Job drawing, mm, ordinate dimensions from the low corner. One solid piece. A direction names the side the tool comes from. Give positions to 0.01 mm unless a question says otherwise; leave off trailing zeros. Order: outer loops, then holes, each group sorted by start corner. A loop starts at its lowest first (then second) coordinate and runs counter-clockwise, first axis right, second up. Notation, with made-up numbers: M -12,14.5 L 37,14.5 A27 cw 37,50.5 Z; hole C 59.5,66 d10. An arc over 180 degrees is marked long. Put each result on its own line as item: value. Start each with the question number.
1) Drill centre lines: line 1 (Z direction, x = 11, y = 0.35); line 2 (Z direction, x = 11, y = 2.25); line 3 (Z direction, x = 13.5, y = 1.75). Where is each one in solid material? Low to high. Write a range as [from, to].
2) Cut at D-D (z = 19). Write the cut outline in (x, y), and give its area (3 significant figures).
3) Tool access for the marked faces 1, 2 and 3: list every direction of +Z, -Z, +X, -X, +Y, -Y with a clear straight run to the whole face (end or side of a thin tool).
4) Pin check, flat tips, straight feed: pin 1 (3 mm diameter, centred on x = 19, y = 3, fed in from -Z); pin 2 (1 mm diameter, centred on x = 5, y = 4, fed in from -Z); pin 3 (9.5 mm diameter, centred on x = 10, z = 7.5, fed in from +Y); pin 4 (4 mm diameter, centred on x = 8, y = 3, fed in from -Z). Stop position of each tip, or through.
5) Two-plate mould, pull along Z, no slides. Class the marked faces 4, 5 and 6: released by +Z, released by -Z, zero draft, split by the parting line, or undercut.
6) Cut at B-B (z = 11). Write the cut outline in (x, y), and give its area (3 significant figures).
7) Cut at A-A (x = 11). Write the cut outline in (y, z), and give its area (3 significant figures).
8) Cut at C-C (y = 4.75). Write the cut outline in (x, z), and give its area (3 significant figures).
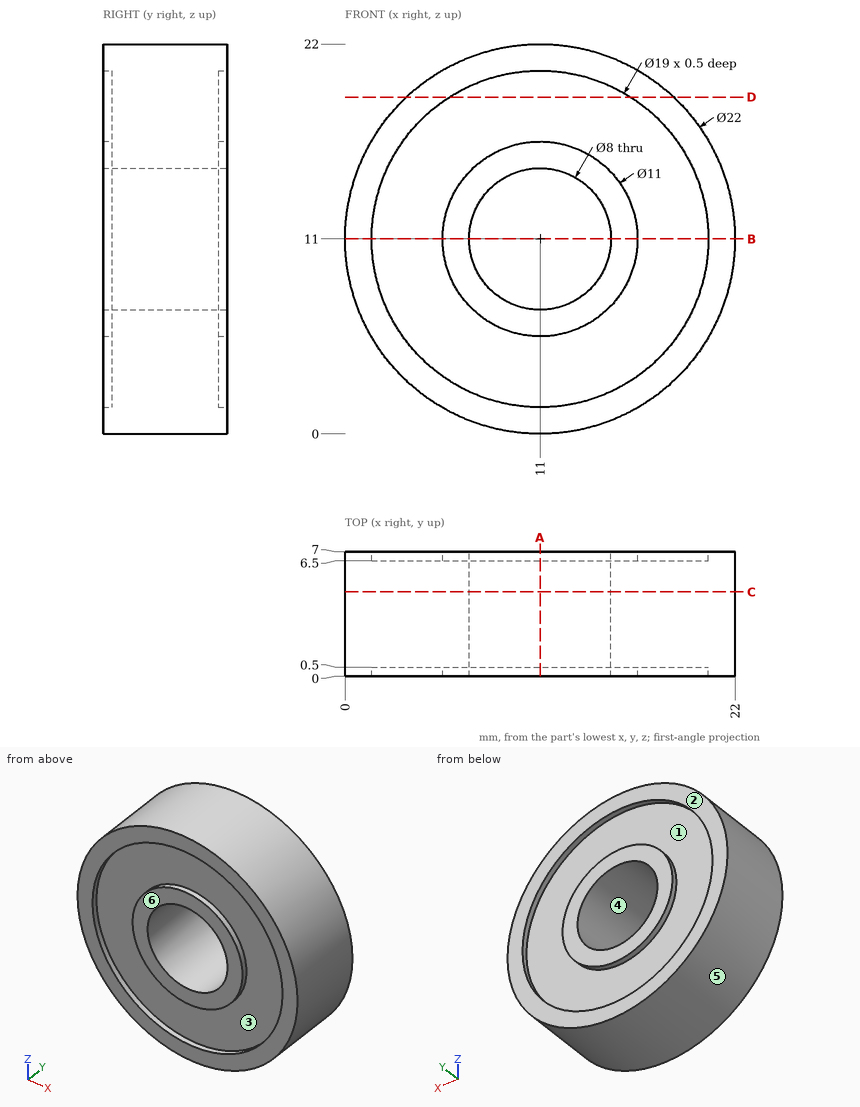
Solution:
1. line 1: [0, 1.5], [5.5, 7], [15, 16.5], [20.5, 22]
1. line 2: [0, 7], [15, 22]
1. line 3: [0.29, 7.88], [14.12, 21.71]
2. outline: M 3.45,0 L 5.88,0 L 5.88,0.5 L 16.12,0.5 L 16.12,0 L 18.55,0 L 18.55,7 L 16.12,7 L 16.12,6.5 L 5.88,6.5 L 5.88,7 L 3.45,7 Z
2. area: 95.5 mm²
3. face 1: +Y
3. face 2: +Z, -Z, +X, -X, +Y
3. face 3: -Y
4. pin 1: z = 2.13
4. pin 2: z = 1.47
4. pin 3: y = 7
4. pin 4: z = 0.05
5. face 4: undercut
5. face 5: split by the parting line
5. face 6: zero draft
6. outline: M 0,0 L 1.5,0 L 1.5,0.5 L 5.5,0.5 L 5.5,0 L 7,0 L 7,7 L 5.5,7 L 5.5,6.5 L 1.5,6.5 L 1.5,7 L 0,7 Z; M 15,0 L 16.5,0 L 16.5,0.5 L 20.5,0.5 L 20.5,0 L 22,0 L 22,7 L 20.5,7 L 20.5,6.5 L 16.5,6.5 L 16.5,7 L 15,7 Z
6. area: 90.0 mm²
7. outline: M 0,0 L 7,0 L 7,1.5 L 6.5,1.5 L 6.5,5.5 L 7,5.5 L 7,7 L 0,7 L 0,5.5 L 0.5,5.5 L 0.5,1.5 L 0,1.5 Z; M 0,15 L 7,15 L 7,16.5 L 6.5,16.5 L 6.5,20.5 L 7,20.5 L 7,22 L 0,22 L 0,20.5 L 0.5,20.5 L 0.5,16.5 L 0,16.5 Z
7. area: 90.0 mm²
8. outline: C 11,11 d22; hole C 11,11 d8
8. area: 330 mm²
